Check sheet for the modelled part. Datum: model origin and axes. Units: mm. Face numbers are marked on the shaded views. Give positions to 0.01 mm unless a question says otherwise; leave off trailing zeros. Loops run counter-clockwise (first coordinate to the right, second up) from the corner with the lowest first, then second, coordinate; pieces in that order, holes last. Notation, with made-up numbers: M 9,4.25 L 63,4.25 A21 cw 63,25.25 Z; hole C 69,69.25 d7. An arc over 180 degrees is marked long. Put each result on its own line as item: value. Start each with the question number.
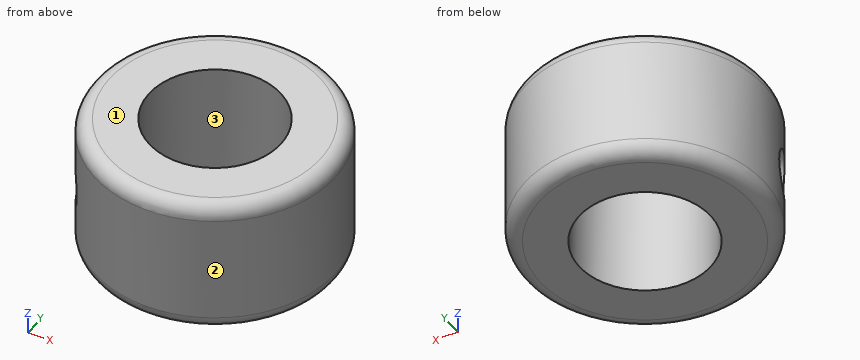
```python
from build123d import *

# Parameters (mm, degrees)
ESQUISSE1_R           = 6.24205
ESQUISSE1_R_2         = 3.429
BOSS_EXTRU_1_DEPTH    = 7.14502
CONG_1_R              = 0.762
D_GAGEMENT_M21_REACH  = 17.35
D_GAGEMENT_M21_BORE_R = 1.3


with BuildPart() as part:
    # Esquisse1 → Boss.-Extru.1 (new body)
    with BuildSketch(Plane.XY):
        with Locations(Location((0, 0, 0), (0, 0, 180))):
            Circle(ESQUISSE1_R)
        with Locations(Location((0, 0, 0), (0, 0, 180))):
            Circle(ESQUISSE1_R_2, mode=Mode.SUBTRACT)
    extrude(amount=BOSS_EXTRU_1_DEPTH)

    # Congé1
    cong_1_edges = [part.edges().sort_by_distance(p)[0] for p in [
        (6.24205, 0, 0),
        (6.24205, 0, 7.14502),
    ]]
    fillet(cong_1_edges, radius=CONG_1_R)

    # Dégagement M21 bore (on position points) → Dégagement M21 (cut, up to next)
    with BuildSketch(Plane(origin=(-5.594728997, -2.768067132, 3.359647544), x_dir=(0.44345481566, -0.896296729029, 0), z_dir=(-0.896296729029, -0.44345481566, 0)), mode=Mode.PRIVATE) as d_gagement_m21_sk1:
        Circle(D_GAGEMENT_M21_BORE_R)
    d_gagement_m21_tool1 = extrude(d_gagement_m21_sk1.sketch, amount=-D_GAGEMENT_M21_REACH, mode=Mode.PRIVATE) & part.part
    add(d_gagement_m21_tool1.solids().sort_by_distance((-5.594729, -2.768067, 3.359648))[0], mode=Mode.SUBTRACT)


solid = part.part
```
Q1. Section check C-C, the plane z = 1.5. Record the cut outline in (x, y).
Q2. Section check A-A, the plane x = 0. Record the cut outline in (y, z).
Q3. Depth check by flat-ended pin: P1, Ø3, axis at x = -1, z = 6, coming from the +Y side; P2, Ø1.5, axis at y = 4.5, z = 4, coming from the -X side; P3, Ø1.5, axis at x = -3.5, z = 1.5, coming from the +Y side; P4, Ø1, axis at x = 1, y = 0.5, coming from the +Z side. Enter the tip coordinate at first touch or a pass-through.
Q4. Section check D-D, the plane z = 2.75. Record the cut outline in (x, y), then the cut area to 3 significant figures.
Q5. Thickness scan on line 1 along Y through (x, z) = (0, 2.5); line 2 along Y through (x, z) = (3, 4.75); line 3 along X through (y, z) = (-1, 2). Record the ranges inside material, lowest first. Write a range as [from, to].
Q6. Mould release check, pull along Y, two halves, no side actions. Record for the marked faces 1, 2 and 3: pulls with the +Y half, pulls with the -Y half, needs draft (parallel to the pull), parting line crosses it, or undercut.
Found:
1. outline: C 0,0 d12.48; hole C 0,0 d6.86
2. outline: M -6.24,0.76 A0.76 ccw -5.48,0 L -3.43,0 L -3.43,7.15 L -5.48,7.15 A0.76 ccw -6.24,6.38 Z; M 3.43,0 L 5.48,0 A0.76 ccw 6.24,0.76 L 6.24,6.38 A0.76 ccw 5.48,7.15 L 3.43,7.15 Z
3. P1: stops at y = 6.24
3. P2: stops at x = -4.99
3. P3: stops at y = 5.6
3. P4: passes through
4. outline: M -6.01,-1.69 L -3.41,-0.4 A3.43 cw long -2.39,-2.46 L -4.99,-3.75 A6.24 ccw long Z
4. area: 78.9 mm^2
5. line 1: y = [-6.24, -3.43], [3.43, 6.24]
5. line 2: y = [-5.47, -1.66], [1.66, 5.47]
5. line 3: x = [-6.16, -3.28], [3.28, 6.16]
6. face 1: needs draft
6. face 2: parting line crosses it
6. face 3: undercut
